```python
from build123d import *

# Parameters (mm, degrees)
ESBO_O2_W             = 15.991560494
ESBO_O2_H             = 5.81194908
CORTE_EXTRUS_O1_DEPTH = 2


with BuildPart() as part:
    # Esboço1 → Revolução1 (revolve)
    with BuildSketch(Plane(origin=(0, 0, 0), x_dir=(0, 0, -1), z_dir=(1, 0, 0))):
        with BuildLine():
            Line((4.220409826, 6.5), (0, 6.5))
            Line((0, 6.5), (0, 5.93167583))
            Line((0, 5.93167583), (0, 4.523660393))
            Line((0, 4.523660393), (3.444296294, 4.523660393))
            Line((3.444296294, 4.523660393), (4.220409826, 4.523660393))
            ThreePointArc((4.220409826, 4.523660393), (7.419120765, 3.198710939), (8.744070218, 0))
            Line((8.744070218, 0), (9.5, 0))
            ThreePointArc((9.5, 0), (7.95364384, 3.733234014), (4.220409826, 5.279590174))
            Line((4.220409826, 5.279590174), (4.220409826, 6.5))
        make_face()
    revolve(axis=Axis((0, 0, 0), (0, 0, -1)))

    # Esboço2 → Corte-extrusão1 (cut)
    with BuildSketch(Plane.XY):
        with Locations((0.060903658, 0.226213587)):
            Rectangle(ESBO_O2_W, ESBO_O2_H)
    extrude(amount=-CORTE_EXTRUS_O1_DEPTH, mode=Mode.SUBTRACT)


solid = part.part
```
Verification items for the finished model (mm, model axes). A direction names the side the tool comes from. Round coordinates to 2 decimals unless told otherwise and drop trailing zeros. Order: outer loops, then holes, each group sorted by start corner. A loop starts at its lowest first (then second) coordinate and runs counter-clockwise, first axis right, second up. Notation, with made-up numbers: (36, -36) -> (79, -36) arc R25 cw to (79, -8) -> close; hole circle Ø1 at (-23.5, 5). An arc over 180 degrees is marked (long way). Put each result on its own line as item: value. Start each with the question number.
(1) Section check A-A (z = -1.25). Enter the section's corners in (x, y).
(2) Material ranges on line 1 along Y through (x, z) = (0, -0.9); line 2 along Z through (x, y) = (5.75, -1), recorded low to high.
(3) Depth check by flat-ended pin: pin 1 Ø1 at (x, y) = (0.5, -3) entering from +Z; pin 2 Ø4 at (x, y) = (-3, -1.5) entering from -Z; pin 3 Ø1 at (x, y) = (4, 1) entering from +Z. Enter the tip coordinate at first touch or a pass-through.
(4) Section check B-B (x = 0). Enter the section's corners in (y, z).
(5) Section check D-D (z = -2.5). Enter the section's corners in (x, y), then the cut area to 3 significant figures.
(6) Section check C-C (y = 0). Enter the section's corners in (x, z), then the cut area to 3 significant figures.
(7) Tool access check on faces 1 (the face through (0.2, -4.52, -2.61)), 2 (the face through (0, -5, 0)), 3 (the face through (-4, 3.132, -1)). Record the directions out of +Z, -Z, +X, -X, +Y, -Y that give a thin tool (end or side, any length) a straight path to the whole face; none if there is none.
Completed:
1. outline: (-5.92, -2.68) arc R6.5 ccw to (5.92, -2.68) -> (3.64, -2.68) arc R4.52 cw to (-3.64, -2.68) -> close; (-5.7, 3.13) -> (-3.26, 3.13) arc R4.52 cw to (3.26, 3.13) -> (5.7, 3.13) arc R6.5 ccw to start
2. line 1: y = -6.5 to -4.52, 4.52 to 6.5
2. line 2: z = -4.22 to -2
3. pin 1: stops at z = -7.04
3. pin 2: stops at z = -9.32
3. pin 3: stops at z = -2
4. outline: (-6.5, -4.22) -> (-5.28, -4.22) arc R5.28 ccw to (5.28, -4.22) -> (6.5, -4.22) -> (6.5, 0) -> (4.52, 0) -> (4.52, -4.22) arc R4.52 cw to (-4.52, -4.22) -> (-4.52, 0) -> (-6.5, 0) -> close
5. outline: circle Ø13 at (0, 0); hole circle Ø9.05 at (0, 0)
5. area: 68.4 mm2
6. outline: (-6.5, -4.22) -> (-5.28, -4.22) arc R5.28 ccw to (5.28, -4.22) -> (6.5, -4.22) -> (6.5, -2) -> (4.52, -2) -> (4.52, -4.22) arc R4.52 cw to (-4.52, -4.22) -> (-4.52, -2) -> (-6.5, -2) -> close
6. area: 20.4 mm2
7. face 1: +Z
7. face 2: +Z, +X, -X, +Y, -Y
7. face 3: +Z, +X, -X
